Build history of the part. All positions in model axes, mm. A direction names the side the tool comes from. Round coordinates to 2 decimals unless told otherwise and drop trailing zeros. Order: outer loops, then holes, each group sorted by start corner. A loop starts at its lowest first (then second) coordinate and runs counter-clockwise, first axis right, second up. Notation, with made-up numbers: M -33.5,44 L 12.5,44 A16 ccw 12.5,61 Z; hole C 21.5,-34 d5. An arc over 180 degrees is marked long. One line per item, written item: value. Start each with the question number.
Item 1: Two-plate mould, pull along Y, no slides. Class faces 3 (the cylindrical face through (0.14, -4.43, 0.6)), 4 (the flat face through (-2.014, 3.104, 3.521)), 5 (the flat face through (-2.4, 3.4, 5)), 6 (the flat face through (0, 0, 2)): +Y half, -Y half, draft (parallel to the pull), parting line (faces both ways), or undercut.
Item 2: Band-saw the part on C-C, the plane x = -4.75. Write the cut outline in (y, z).
Item 3: Pin check, flat tip, straight feed: pin 1 (3 mm diameter, centred on x = 1.5, y = 0, fed in from +Z). Stop position of the tip, or through.
Item 4: Tool access for faces 1 (the flat face through (0, 0, 0)), 2 (the flat face through (2.014, -3.104, 3.521)): list every direction of +Z, -Z, +X, -X, +Y, -Y with a clear straight run to the whole face (end or side of a thin tool).
Item 5: Band-saw the part on D-D, the plane y = -2.75. Write the cut outline in (x, z).
Item 6: Band-saw the part on B-B, the plane y = -1. Write the cut outline in (x, z), then the cut area to 3 significant figures.
Item 7: Probe L1, parallel to Z at x = 0, y = -0.25; L2, parallel to X at y = -4, z = 1.9; L3, parallel to X at y = -4, z = 2.75. List the from-to ranges inside material, lowest first.
Item 8: Band-saw the part on A-A, the plane z = 4.75. Write the cut outline in (x, y), then the cut area to 3 significant figures.
```python
from build123d import *

# Parameters (mm, degrees)
SKETCH1_W           = 20
SKETCH1_H           = 10
BOSS_EXTRUDE1_DEPTH = 5
CUT_EXTRUDE1_DEPTH  = 3
FILLET1_R           = 2


with BuildPart() as part:
    # Sketch1 → Boss-Extrude1 (new body)
    with BuildSketch(Plane.XY):
        Rectangle(SKETCH1_W, SKETCH1_H)
    extrude(amount=BOSS_EXTRUDE1_DEPTH)

    # Sketch2 → Cut-Extrude1 (cut)
    with BuildSketch(Plane.XY.offset(5)):
        Polygon((0.255981481, -4.264716499), (3.821343568, -1.910671784), (3.565362087, 2.354044715), (-0.255981481, 4.264716499), (-3.821343568, 1.910671784), (-3.565362087, -2.354044715), align=None)
    extrude(amount=-CUT_EXTRUDE1_DEPTH, mode=Mode.SUBTRACT)

    # Fillet1
    fillet1_edges = [part.edges().sort_by_distance(p)[0] for p in [
        (0, -5, 0),
        (-10, 0, 0),
        (0, 5, 0),
        (10, 0, 0),
    ]]
    fillet(fillet1_edges, radius=FILLET1_R)


solid = part.part
```
Output:
1. face 3: -Y half
1. face 4: undercut
1. face 5: draft
1. face 6: undercut
2. outline: M -5,2 A2 ccw -3,0 L 3,0 A2 ccw 5,2 L 5,5 L -5,5 Z
3. pin 1: stops at z = 2
4. face 1: -Z, +X, -X, +Y, -Y
4. face 2: +Z
5. outline: M -10,2 A2 ccw -8,0 L 8,0 A2 ccw 10,2 L 10,5 L 2.55,5 L 2.55,2 L -2.77,2 L -2.77,5 L -10,5 Z
6. outline: M -10,2 A2 ccw -8,0 L 8,0 A2 ccw 10,2 L 10,5 L 3.77,5 L 3.77,2 L -3.65,2 L -3.65,5 L -10,5 Z
6. area: 76.0 mm²
7. L1: z = 0 to 2
7. L2: x = -10 to 10
7. L3: x = -10 to -0.27, 0.66 to 10
8. outline: M -10,-5 L 10,-5 L 10,5 L -10,5 Z; hole M -3.82,1.91 L -3.57,-2.35 L 0.26,-4.26 L 3.82,-1.91 L 3.57,2.35 L -0.26,4.26 Z
8. area: 153 mm²
